Verification items for the finished model (mm, model axes). Face numbers are marked on the shaded views. A direction names the side the tool comes from. Round coordinates to 2 decimals unless told otherwise and drop trailing zeros. Loops run counter-clockwise (first coordinate to the right, second up) from the corner with the lowest first, then second, coordinate; pieces in that order, holes last. Notation, with made-up numbers: M 17.25,77 L 44.25,77 A21 ccw 44.25,93 Z; hole C -24,41 d4. An arc over 180 degrees is marked long. Answer as CSV lines item,"result".
```python
from build123d import *

# Parameters (mm, degrees)
SKETCH1_R           = 1.6
BOSS_EXTRUDE1_DEPTH = 5
BOSS_EXTRUDE5_DEPTH = 20
FILLET8_R           = 34
FILLET9_R           = 37
REVOLVE4_ANGLE      = 90
BOSS_EXTRUDE6_DEPTH = 20
CUT_EXTRUDE3_REACH  = 593.738
SKETCH16_W          = 40
SKETCH16_H          = 5
FILLET10_R          = 22
CUT_EXTRUDE4_REACH  = 581.899
SKETCH17_R          = 7.5
FILLET11_R          = 5
FILLET12_R          = 2
SKETCH18_R          = 3
CUT_EXTRUDE5_DEPTH  = 7


with BuildPart() as part:
    # Sketch1 → Boss-Extrude1 (new body)
    with BuildSketch(Plane(origin=(0, 0, 0), x_dir=(1, 0, 0), z_dir=(0, 1, 0))):
        Polygon((-165, 270), (-165, -270), (0, -270), (0, -254), (-149, -254), (-149, 254), (0, 254), (0, 270), align=None)
        with Locations(Location((-159, 130, 0), (0, 0, 270))):
            Circle(SKETCH1_R, mode=Mode.SUBTRACT)
        with Locations(Location((-159, 50, 0), (0, 0, 270))):
            Circle(SKETCH1_R, mode=Mode.SUBTRACT)
        with Locations(Location((-120, 264, 0), (0, 0, 270))):
            Circle(SKETCH1_R, mode=Mode.SUBTRACT)
        with Locations(Location((-40, 264, 0), (0, 0, 270))):
            Circle(SKETCH1_R, mode=Mode.SUBTRACT)
        with Locations(Location((-159, 210, 0), (0, 0, 270))):
            Circle(SKETCH1_R, mode=Mode.SUBTRACT)
        with Locations(Location((-40, -264, 0), (0, 0, 90))):
            Circle(SKETCH1_R, mode=Mode.SUBTRACT)
        with Locations(Location((-120, -264, 0), (0, 0, 90))):
            Circle(SKETCH1_R, mode=Mode.SUBTRACT)
        with Locations(Location((-159, -210, 0), (0, 0, 90))):
            Circle(SKETCH1_R, mode=Mode.SUBTRACT)
        with Locations(Location((-159, -50, 0), (0, 0, 90))):
            Circle(SKETCH1_R, mode=Mode.SUBTRACT)
        with Locations(Location((-159, -130, 0), (0, 0, 90))):
            Circle(SKETCH1_R, mode=Mode.SUBTRACT)
    extrude(amount=BOSS_EXTRUDE1_DEPTH)

    # Sketch12 → Boss-Extrude5 (add)
    with BuildSketch(Plane(origin=(0, 5, 0), x_dir=(1, 0, 0), z_dir=(0, 1, 0))):
        Polygon((0, 254), (-149, 254), (-149, -254), (0, -254), (0, -257), (-152, -257), (-152, 257), (0, 257), align=None)
    extrude(amount=BOSS_EXTRUDE5_DEPTH)

    # Fillet8
    fillet8_edges = [part.edges().sort_by_distance(p)[0] for p in [
        (-149, 12.5, -254),
        (-149, 12.5, 254),
    ]]
    fillet(fillet8_edges, radius=FILLET8_R)

    # Fillet9
    fillet9_edges = [part.edges().sort_by_distance(p)[0] for p in [
        (-152, 15, -257),
        (-152, 15, 257),
    ]]
    fillet(fillet9_edges, radius=FILLET9_R)

    # Sketch13 → Revolve4 (revolve)
    with BuildSketch(Plane(origin=(0, 25, 0), x_dir=(1, 0, 0), z_dir=(0, 1, 0))):
        with BuildLine():
            Line((0, 254), (-115, 254))
            ThreePointArc((-115, 254), (-139.04163056, 244.04163056), (-149, 220))
            Line((-149, 220), (-149, -220))
            ThreePointArc((-149, -220), (-139.04163056, -244.04163056), (-115, -254))
            Line((-115, -254), (0, -254))
            Line((0, -254), (0, -257))
            Line((0, -257), (-115, -257))
            ThreePointArc((-115, -257), (-141.162950904, -246.162950904), (-152, -220))
            Line((-152, -220), (-152, 220))
            ThreePointArc((-152, 220), (-141.162950904, 246.162950904), (-115, 257))
            Line((-115, 257), (0, 257))
            Line((0, 257), (0, 254))
        make_face()
    revolve(axis=Axis((0, 25, -257), (0, 0, -1)), revolution_arc=REVOLVE4_ANGLE)

    # Sketch15 → Boss-Extrude6 (add)
    with BuildSketch(Plane(origin=(0, 0, 0), x_dir=(0, 0, -1), z_dir=(1, 0, 0))):
        with BuildLine():
            Line((-254, 5), (-254, 140))
            ThreePointArc((-254, 140), (-244.04163056, 164.04163056), (-220, 174))
            Line((-220, 174), (220, 174))
            ThreePointArc((220, 174), (244.04163056, 164.04163056), (254, 140))
            Line((254, 140), (254, 5))
            Line((254, 5), (254, 0))
            Line((254, 0), (270, 0))
            Line((270, 0), (270, 5))
            Line((270, 5), (257, 5))
            Line((257, 5), (257, 140))
            ThreePointArc((257, 140), (246.162950904, 166.162950904), (220, 177))
            Line((220, 177), (-220, 177))
            ThreePointArc((-220, 177), (-246.162950904, 166.162950904), (-257, 140))
            Line((-257, 140), (-257, 5))
            Line((-257, 5), (-270, 5))
            Line((-270, 5), (-270, 0))
            Line((-270, 0), (-254, 0))
            Line((-254, 0), (-254, 5))
        make_face()
    extrude(amount=BOSS_EXTRUDE6_DEPTH)

    # Cut-Extrude3: up to this face of the body (flat: up to its plane)
    cut_extrude3_end = Plane(part.part.faces().sort_by_distance((-72.5, 2.5, -270))[0])
    # Sketch16 → Cut-Extrude3 (cut, up to the picked face)
    with BuildSketch(Plane.XY.offset(270), mode=Mode.PRIVATE) as cut_extrude3_sk1:
        with Locations((0, 2.5)):
            Rectangle(SKETCH16_W, SKETCH16_H)
    cut_extrude3_tool1 = split(extrude(cut_extrude3_sk1.sketch, amount=-CUT_EXTRUDE3_REACH, mode=Mode.PRIVATE), bisect_by=cut_extrude3_end, keep=Keep.BOTH, mode=Mode.PRIVATE)
    add(cut_extrude3_tool1.solids().sort_by(Axis((0, 2.5, 270), (0, 0, -1)))[0], mode=Mode.SUBTRACT)

    # Fillet10
    fillet10_edges = [part.edges().sort_by_distance(p)[0] for p in [
        (20, 5, 255.5),
        (20, 5, -255.5),
    ]]
    fillet(fillet10_edges, radius=FILLET10_R)

    # Cut-Extrude4: up to this face of the body (flat: up to its plane)
    cut_extrude4_end = Plane(part.part.faces().sort_by_distance((-40.16059182, 65.16059182, -257))[0])
    # Sketch17 → Cut-Extrude4 (cut, up to the picked face)
    with BuildSketch(Plane.XY.offset(257), mode=Mode.PRIVATE) as cut_extrude4_sk1:
        with Locations((0, 25)):
            Circle(SKETCH17_R)
    cut_extrude4_tool1 = split(extrude(cut_extrude4_sk1.sketch, amount=-CUT_EXTRUDE4_REACH, mode=Mode.PRIVATE), bisect_by=cut_extrude4_end, keep=Keep.BOTH, mode=Mode.PRIVATE)
    add(cut_extrude4_tool1.solids().sort_by(Axis((0, 25, 257), (0, 0, -1)))[0], mode=Mode.SUBTRACT)

    # Fillet11
    fillet11_edges = [part.edges().sort_by_distance(p)[0] for p in [
        (-165, 2.5, 270),
        (-165, 2.5, -270),
    ]]
    fillet(fillet11_edges, radius=FILLET11_R)

    # Fillet12
    fillet12_edges = [part.edges().sort_by_distance(p)[0] for p in [
        (-152, 5, 0),
        (-67.5, 5, 257),
        (-141.162950904, 5, -246.162950904),
        (-141.162950904, 5, 246.162950904),
        (-67.5, 5, -257),
    ]]
    fillet(fillet12_edges, radius=FILLET12_R)

    # Sketch18 → Cut-Extrude5 (cut)
    with BuildSketch(Plane(origin=(0, 0, -257), x_dir=(-1, 0, 0), z_dir=(0, 0, -1))):
        with Locations((99.306112319, 13.240065646)):
            Circle(SKETCH18_R)
    extrude(amount=-CUT_EXTRUDE5_DEPTH, mode=Mode.SUBTRACT)


solid = part.part
```
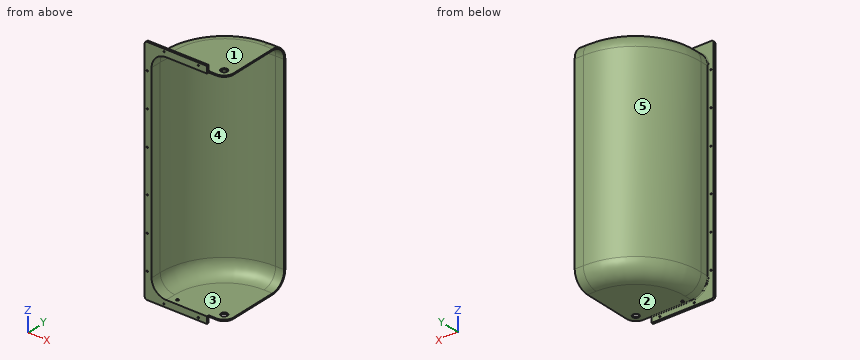
1) Material ranges on probe 1 along X at (y, z) = (3.5, 264); probe 2 along Z at (x, y) = (-101, 66); probe 3 along X at (y, z) = (2, -130), recorded low to high.
Here are the results:
probe 1,"x = -165 to -121.6, -118.4 to -41.6, -38.4 to -20"
probe 2,"z = -257 to -254, 254 to 257"
probe 3,"x = -165 to -160.6, -157.4 to -149"
2) Draft check along Z on the marked faces 1, 2 and 3. Enter one of: +Z half, -Z half, draft (parallel to the pull), parting line (faces both ways), or undercut.
Here are the results:
face 1,"+Z half"
face 2,"-Z half"
face 3,"undercut"
3) Set-up check for the marked faces 4 and 5: record each of +Z, -Z, +X, -X, +Y, -Y from which the full face is reachable in a straight line by a thin tool's end or side.
Here are the results:
face 4,"+X, -Y"
face 5,"+Z, -Z, -X, +Y"
4) Go/stop test with flat-tipped pins: pin 1 (6 mm diameter, centred on y = 111, z = -142, fed in from +X); pin 2 (8 mm diameter, centred on y = 90, z = -178, fed in from +X); pin 3 (4 mm diameter, centred on x = -159, z = -210, fed in from +Y). Record where each tip stops, or that it passes through.
Here are the results:
pin 1,"stops at x = -119.5"
pin 2,"stops at x = -132.06"
pin 3,"stops at y = 5"
5) Section check A-A (z = 147.5). Record the cut outline in (x, y).
Here are the results:
outline,"M -165,0 L -149,0 L -149,25 A149 cw 0,174 L 20,174 L 20,177 L 0,177 A152 ccw -152,25 L -152,7 A2 cw -154,5 L -165,5 Z"
